Here's the drawing with two shaded views (mm, measured from the low corner). I have some questions. A direction names the side the tool comes from. Coordinates: 2 decimals unless noted, no trailing zeros. Write each loop counter-clockwise with the first axis right and the second up, starting at its lowest first coordinate (ties: lowest second). Pieces come first, ordered by that corner, then holes. Notation, with made-up numbers: M 57,-9.75 L 66,-9.75 A26 ccw 66,8.25 Z; hole C -6.5,83.25 d10. An arc over 180 degrees is marked long. Answer as CSV lines item,"result". Start each with the question number.
Item 1: Suppose I cut it at D-D, the plane y = 25.4. Write out the boundary of the cut face in (x, z) (1 decimal).
Item 2: We'd pull the mould along Z, two halves only. Please class the marked faces 1, 2, 3 and 4: +Z half, -Z half, draft (parallel to the pull), parting line (faces both ways), or undercut.
Item 3: Suppose I cut it at C-C, the plane x = 19. Write out the boundary of the cut face in (y, z) (3 decimals).
Item 4: Suppose I cut it at B-B, the plane z = 2. Write out the boundary of the cut face in (x, y) (1 decimal), and give its area (3 significant figures).
Item 5: Suppose I cut it at A-A, the plane x = 38.1. Write out the boundary of the cut face in (y, z) (1 decimal).
Item 6: I'm going to push flat-ended pins straight in: P1, Ø5, axis at y = 22.5, z = 17.5, coming from the +X side (3 decimals); P2, Ø2.5, axis at x = 35, z = 23, coming from the -Y side; P3, Ø1, axis at x = 27.5, z = 4.5, coming from the -Y side; P4, Ø1, axis at x = 8, z = 22.5, coming from the +Y side. Where does each tip first touch, or does it pass through?
Item 7: If I drill on line 1 along Y through (x, z) = (38.1, 24.1); line 2 along Z through (x, y) = (46, 30) (3 decimals); line 3 along Y through (x, z) = (11, 23.5), over which ranges is the centre line in solid material (lowest first)? Write a range as [from, to].
Item 8: On a 3-axis mill with a long thin cutter (end or side, diameter ignored), from which of +Z, -Z, +X, -X, +Y, -Y can I reach the whole of each face in a straight line? I mean the marked faces 5 and 6. Say none if no direction works.
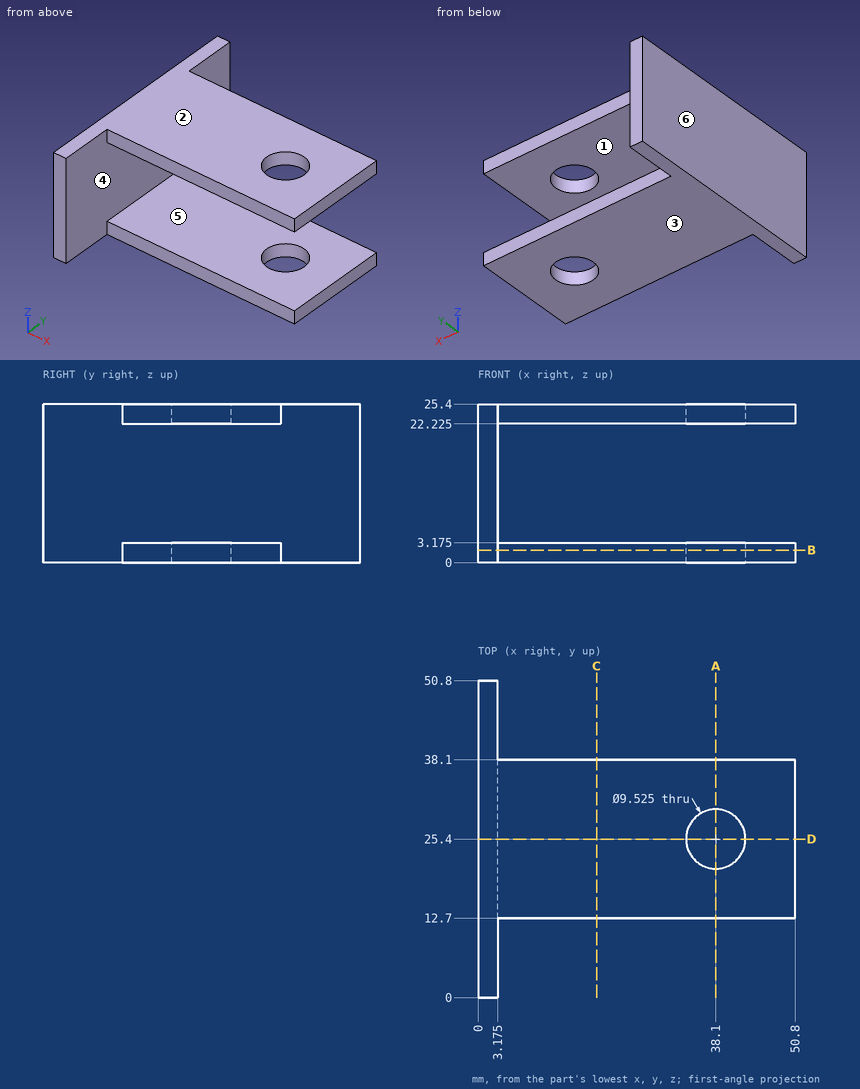
Ans:
1,outline,"M 0,0 L 33.3,0 L 33.3,3.2 L 3.2,3.2 L 3.2,22.2 L 33.3,22.2 L 33.3,25.4 L 0,25.4 Z; M 42.9,0 L 50.8,0 L 50.8,3.2 L 42.9,3.2 Z; M 42.9,22.2 L 50.8,22.2 L 50.8,25.4 L 42.9,25.4 Z"
2,face 1,"undercut"
2,face 2,"+Z half"
2,face 3,"-Z half"
2,face 4,"undercut"
3,outline,"M 12.7,0 L 38.1,0 L 38.1,3.175 L 12.7,3.175 Z; M 12.7,22.225 L 38.1,22.225 L 38.1,25.4 L 12.7,25.4 Z"
4,outline,"M 0,0 L 3.2,0 L 3.2,12.7 L 50.8,12.7 L 50.8,38.1 L 3.2,38.1 L 3.2,50.8 L 0,50.8 Z; hole C 38.1,25.4 d9.5"
4,area,"1,300 mm^2"
5,outline,"M 12.7,0 L 20.6,0 L 20.6,3.2 L 12.7,3.2 Z; M 12.7,22.2 L 20.6,22.2 L 20.6,25.4 L 12.7,25.4 Z; M 30.2,0 L 38.1,0 L 38.1,3.2 L 30.2,3.2 Z; M 30.2,22.2 L 38.1,22.2 L 38.1,25.4 L 30.2,25.4 Z"
6,P1,"stops at x = 3.175"
6,P2,"stops at y = 12.7"
6,P3,"passes through"
6,P4,"stops at y = 38.1"
7,line 1,"y = [12.7, 20.64], [30.16, 38.1]"
7,line 2,"z = [0, 3.175], [22.225, 25.4]"
7,line 3,"y = [12.7, 38.1]"
8,face 5,"+X, +Y, -Y"
8,face 6,"+Z, -Z, -X, +Y, -Y"
